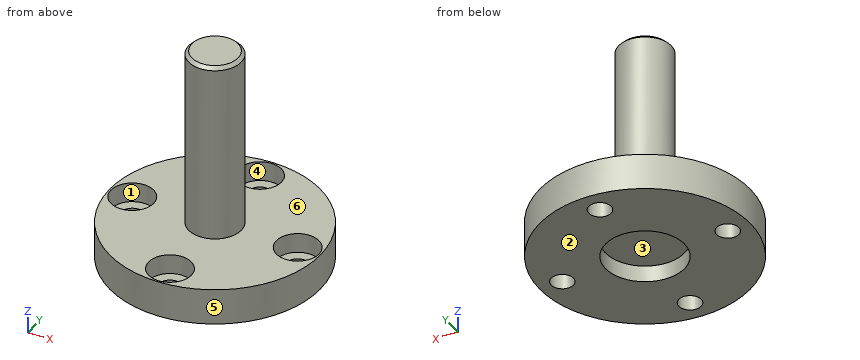
Autodesk Inventor part; units mm, degrees
ref_plane "YZ Plane" through (0, 0, 0) normal (1, 0, 0) x (0, 1, 0)
ref_plane "XZ Plane" through (0, 0, 0) normal (0, 1, 0) x (-1, 0, 0)
ref_plane "XY Plane" through (0, 0, 0) normal (0, 0, 1) x (1, 0, 0)
sketch "スケッチ1" plane through (0, 0, 0) normal (1, 0, 0) x (0, 1, 0)
  line L0 (0, 33) -> (4, 33)
  line L1 (4, 33) -> (4, 5.5)
  line L2 (4, 5.5) -> (16, 5.5)
  line L3 (16, 5.5) -> (16, 0)
  line L4 (0, 33) -> (0, 2.5)
  line L5 (0, 2.5) -> (6, 2.5)
  line L6 (6, 2.5) -> (6, 0)
  line L7 (6, 0) -> (16, 0)
  point P0 (0, 0)
  dimension "d0" = 4
  dimension "d2" = 5.5
  dimension "d3" = 27.5
  dimension "d22" = 2.5
  dimension "d23" = 6
  dimension "d24" = 16
revolve "回転1" add sketch "スケッチ1" angle 360 about axis through (0, 0, 33) along (0, 0, -1)
sketch "スケッチ2" plane through (0, 0, 5.5) normal (0, 0, 1) x (1, 0, 0)
  circle A0 centre (0, 0) radius 12.5
  point P0 (0, 0)
  point P1 (0, 12.5)
  point P2 (-12.5, 0)
  point P3 (0, -12.5)
  point P4 (12.5, 0)
  dimension "d5" = 25
  dimension "d8" = 360
hole "穴1" at (0, 12.5, 5.5) at (-12.5, 0, 5.5) at (0, -12.5, 5.5) at (12.5, 0, 5.5) direction (0, 0, -1) diameter 3.4 end through all counterbore diameter 6.5 counterbore depth 3
thread "ねじ1"
chamfer "面取り1" distance 0.5 angle 45 1 edges at (0, -4, 33)
properties part number "adapter1" material "アルミニウム 6061"
Here's how the part is built. I have some questions about the finished solid (model axes, mm). Face numbers are marked on the shaded views. A direction names the side the tool comes from. Coordinates: 2 decimals unless noted, no trailing zeros. Order: outer loops, then holes, each group sorted by start corner. A loop starts at its lowest first (then second) coordinate and runs counter-clockwise, first axis right, second up. Notation, with made-up numbers: (87.5, 79) - (99.5, 79) arc R22 ccw to (99.5, 113) - close; hole circle Ø11 at (15.25, 26.5). An arc over 180 degrees is marked (long way). Use CSV: the item, a comma, the result in double quotes. Start each with the question number.
1. Please list where these lines run through material, in increasing order: line 1 (X direction, y = 0, z = 4); line 2 (Z direction, x = -4.5, y = -11.5); line 3 (Z direction, x = 12.5, y = 2). Write a range as from..to.
2. For the marked faces 1, 2 and 3, which set-ups out of +Z, -Z, +X, -X, +Y, -Y let a thin tool reach every point of the face, with its end or its side?
3. Suppose I cut it at D-D on x = 12.5. List the corners of the cut face in (y, z) for me.
4. Suppose I cut it at C-C on y = -13. List the corners of the cut face in (x, z) for me, then the cut area to 3 significant figures.
5. I'm going to push flat-ended pins straight in: pin 1 (12 mm diameter, centred on x = 6.5, z = 28.5, fed in from +Y); pin 2 (3 mm diameter, centred on y = -3.5, z = 25, fed in from -X); pin 3 (10 mm diameter, centred on y = 7.5, z = 19.5, fed in from +X); pin 4 (2.5 mm diameter, centred on x = 0, y = -12.5, fed in from +Z). Where does each tip first touch, or does it pass through?
6. Suppose I cut it at A-A on y = 0. Give the number of separate pieces and of enclosed holes in the cut face, then the cut area to 3 significant figures.
7. If we mould it in two halves opening along Y, with no side actions, what happens to the marked faces 4, 5 and 6? For each: +Y half, -Y half, draft (parallel to the pull), parting line (faces both ways), or undercut.
Output:
1,line 1,"x = -16..-15.75, -9.25..9.25, 15.75..16"
1,line 2,"z = 0..5.5"
1,line 3,"z = 0..2.5"
2,face 1,"+Z"
2,face 2,"-Z, +X, -X, +Y, -Y"
2,face 3,"-Z"
3,outline,"(-9.99, 0) - (-1.7, 0) - (-1.7, 2.5) - (-3.25, 2.5) - (-3.25, 5.5) - (-9.99, 5.5) - close; (1.7, 0) - (9.99, 0) - (9.99, 5.5) - (3.25, 5.5) - (3.25, 2.5) - (1.7, 2.5) - close"
4,outline,"(-9.33, 0) - (-1.62, 0) - (-1.62, 2.5) - (-3.21, 2.5) - (-3.21, 5.5) - (-9.33, 5.5) - close; (1.62, 0) - (9.33, 0) - (9.33, 5.5) - (3.21, 5.5) - (3.21, 2.5) - (1.62, 2.5) - close"
4,area,"75.2 mm2"
5,pin 1,"stops at y = 3.97"
5,pin 2,"stops at x = -3.46"
5,pin 3,"stops at x = 3.12"
5,pin 4,"passes through"
6,separate pieces,"3"
6,enclosed holes,"0"
6,area,"310 mm2"
7,face 4,"undercut"
7,face 5,"parting line"
7,face 6,"draft"
